Build history of the part. All positions in model axes, mm. Give positions to 0.01 mm unless a question says otherwise; leave off trailing zeros. Order: outer loops, then holes, each group sorted by start corner. A loop starts at its lowest first (then second) coordinate and runs counter-clockwise, first axis right, second up. Notation, with made-up numbers: (56, 16.5) - (61, 16.5) arc R36 ccw to (61, 55.5) - close; hole circle Ø3 at (25, 62). An arc over 180 degrees is marked (long way). One line per item, written item: value.
```python
from build123d import *

# Parameters (mm, degrees)
SKETCH4_R           = 8
SKETCH4_W           = 12.4
SKETCH4_H           = 22.6
BOSS_EXTRUDE2_DEPTH = 3


with BuildPart() as part:
    # Sketch4 → Boss-Extrude2 (new body)
    with BuildSketch(Plane(origin=(0, 0, 0), x_dir=(1, 0, 0), z_dir=(0, 1, 0))):
        Polygon((-26, -90), (-9.5, -90), (-9.5, -87), (15.5, -87), (15.5, -90), (32, -90), (32, -78), (29, -78), (29, -56), (32, -56), (32, -34), (29, -34), (29, -12), (32, -12), (32, 0), (15.5, 0), (15.5, -3), (-9.5, -3), (-9.5, 0), (-26, 0), (-26, -12), (-23, -12), (-23, -34), (-26, -34), (-26, -56), (-23, -56), (-23, -78), (-26, -78), align=None)
        with Locations((12.802419237, -37.2)):
            Circle(SKETCH4_R, mode=Mode.SUBTRACT)
        with Locations((-12, -50)):
            Rectangle(SKETCH4_W, SKETCH4_H, mode=Mode.SUBTRACT)
    extrude(amount=BOSS_EXTRUDE2_DEPTH)


solid = part.part
```
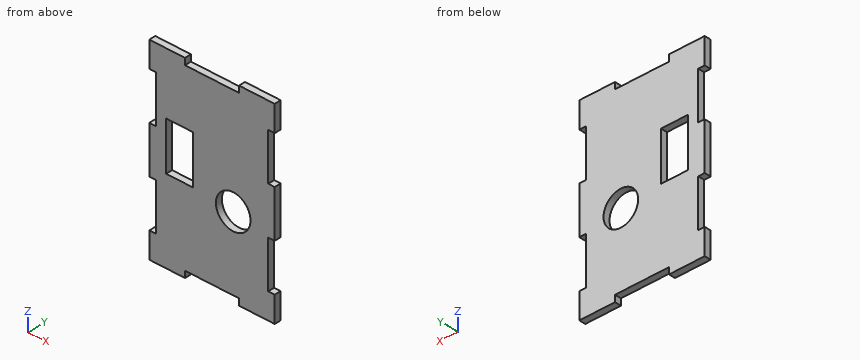
(1) Slice it at A-A, the plane z = 37.2. Give the cut face in (x, y), and give its area (3 significant figures).
Completed:
outline: (-26, 0) - (4.8, 0) - (4.8, 3) - (-26, 3) - close; (20.8, 0) - (32, 0) - (32, 3) - (20.8, 3) - close
area: 126 mm²
(2) Slice it at C-C, the plane y = 2.3. Count the separate pieces of the cut face and the enclosed holes in it, and give its area (3 significant figures).
Completed:
separate pieces: 1
enclosed holes: 2
area: 4,320 mm²
(3) Slice it at D-D, the plane z = 65.5. Give the cut face in (x, y), and give its area (3 significant figures).
Completed:
outline: (-23, 0) - (29, 0) - (29, 3) - (-23, 3) - close
area: 156 mm²
(4) Drill centre lines: line 1 (Z direction, x = -9, y = 1.1); line 2 (Z direction, x = -14, y = 1.85); line 3 (X direction, y = 1.85, z = 37.2). Where is each one in solid material? Low to high.
Completed:
line 1: 3 to 38.7, 61.3 to 87
line 2: 0 to 38.7, 61.3 to 90
line 3: -26 to 4.8, 20.8 to 32
(5) Slice it at B-B, the plane x = -11. Give the cut face in (y, z), and give its area (3 significant figures).
Completed:
outline: (0, 0) - (3, 0) - (3, 38.7) - (0, 38.7) - close; (0, 61.3) - (3, 61.3) - (3, 90) - (0, 90) - close
area: 202 mm²
